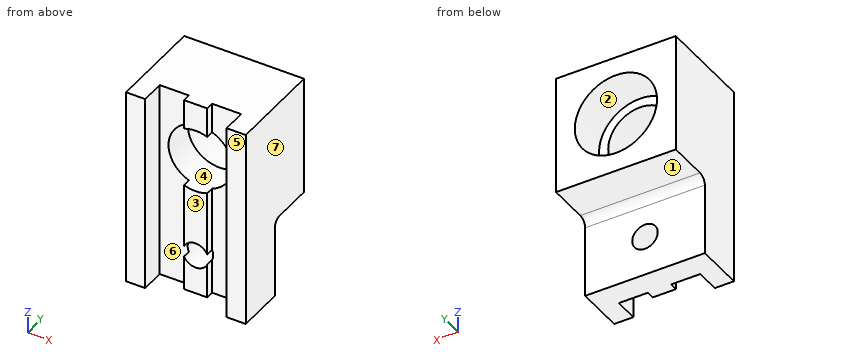
from build123d import *

# Parameters (mm, degrees)
MAIN_DEPTH         = 25
SKETCH2_R          = 5.15
ROLLINGHOLE_DEPTH  = 5
SKETCH3_R          = 4
CUT_EXTRUDE2_DEPTH = 8
SKETCH4_R          = 1.6
FIXHOLE_DEPTH      = 13
SKETCH5_W          = 10
SKETCH5_H          = 6
CUT_EXTRUDE4_DEPTH = 16
FILLET1_R          = 1


with BuildPart() as part:
    # Sketch1 → Main (new body)
    with BuildSketch(Plane.XY):
        Polygon((-5.1, 0), (-5.1, -3), (-7.5, -3), (-7.5, 9), (7.5, 9), (7.5, -3), (5.1, -3), (5.1, 0), (1.45, 0), (1.45, -1), (-1.45, -1), (-1.45, 0), align=None)
    extrude(amount=MAIN_DEPTH)

    # Sketch2 → RollingHole (cut)
    with BuildSketch(Plane(origin=(0, 9, 0), x_dir=(1, 0, 0), z_dir=(0, 1, 0))):
        with Locations((0, -17.5)):
            Circle(SKETCH2_R)
    extrude(amount=-ROLLINGHOLE_DEPTH, mode=Mode.SUBTRACT)

    # Sketch3 → Cut-Extrude2 (cut, through all)
    with BuildSketch(Plane(origin=(0, 4, 0), x_dir=(1, 0, 0), z_dir=(0, 1, 0))):
        with Locations((0, -17.5)):
            Circle(SKETCH3_R)
    extrude(amount=-CUT_EXTRUDE2_DEPTH, mode=Mode.SUBTRACT)

    # Sketch4 → FixHole (cut, through all)
    with BuildSketch(Plane(origin=(0, 9, 0), x_dir=(1, 0, 0), z_dir=(0, 1, 0))):
        with Locations((0, -5)):
            Circle(SKETCH4_R)
    extrude(amount=-FIXHOLE_DEPTH, mode=Mode.SUBTRACT)

    # Sketch5 → Cut-Extrude4 (cut, through all)
    with BuildSketch(Plane.ZY.offset(7.5)):
        with Locations((5, 6)):
            Rectangle(SKETCH5_W, SKETCH5_H)
    extrude(amount=-CUT_EXTRUDE4_DEPTH, mode=Mode.SUBTRACT)

    # Fillet1
    fillet1_edges = [part.edges().sort_by_distance(p)[0] for p in [
        (0, 3, 10),
    ]]
    fillet(fillet1_edges, radius=FILLET1_R)


solid = part.part
Check sheet for the modelled part. Datum: model origin and axes. Units: mm. Face numbers are marked on the shaded views. A direction names the side the tool comes from. Round coordinates to 2 decimals unless told otherwise and drop trailing zeros. Order: outer loops, then holes, each group sorted by start corner. A loop starts at its lowest first (then second) coordinate and runs counter-clockwise, first axis right, second up. Notation, with made-up numbers: M -33.5,19 L 8.5,19 A25 cw 8.5,45 Z; hole C 4,85.5 d2. An arc over 180 degrees is marked long. One line per item, written item: value. Start each with the question number.
1. Section check C-C on x = 0. Enter the section's corners in (y, z), and give its area (3 significant figures).
2. Access from +Z, -Z, +X, -X, +Y, -Y to the whole of each face (thin tool, end or side, straight path). Record for the marked faces 1, 2, 3 and 4.
3. Section check B-B on z = 17.5. Enter the section's corners in (x, y).
4. Release check for a two-part mould opening along X. For the marked faces 5, 6 and 7 record: released by +X, released by -X, zero draft, split by the parting line, or undercut.
5. Section check D-D on y = 6.5. Enter the section's corners in (x, z).
6. Section check A-A on y = -0.5. Enter the section's corners in (x, z).
7. Gauge pin test, flat ends, axial feed: P1, Ø1.5, axis at x = 0, z = 22.5, coming from the -Y side; P2, Ø1.5, axis at x = -4.5, z = 9, coming from the +Y side; P3, Ø4, axis at x = 0, z = 5, coming from the +Y side. Record the tip position at first contact, or that the pin passes through.
8. Scan lines: line 1 along Z through (x, y) = (0, 0.6); line 2 along X through (y, z) = (0.4, 5); line 3 along X through (y, z) = (2.65, 17.5). Record each from-to range of solid material in increasing order.
Results found:
1. outline: M -1,0 L 3,0 L 3,3.4 L -1,3.4 Z; M -1,6.6 L 3,6.6 L 3,9 A1 cw 4,10 L 9,10 L 9,12.35 L 4,12.35 L 4,13.5 L -1,13.5 Z; M -1,21.5 L 4,21.5 L 4,22.65 L 9,22.65 L 9,25 L -1,25 Z
1. area: 85.9 mm^2
2. face 1: -Z, +X, -X, +Y
2. face 2: +Y
2. face 3: +Z, -Z, -Y
2. face 4: +Y, -Y
3. outline: M -7.5,-3 L -5.1,-3 L -5.1,0 L -4,0 L -4,4 L -5.15,4 L -5.15,9 L -7.5,9 Z; M 4,0 L 5.1,0 L 5.1,-3 L 7.5,-3 L 7.5,9 L 5.15,9 L 5.15,4 L 4,4 Z
4. face 5: zero draft
4. face 6: undercut
4. face 7: released by +X
5. outline: M -7.5,10 L 7.5,10 L 7.5,25 L -7.5,25 Z; hole C 0,17.5 d10.3
6. outline: M -7.5,0 L -5.1,0 L -5.1,25 L -7.5,25 Z; M -1.45,0 L 1.45,0 L 1.45,4.32 A1.6 cw -1.45,4.32 Z; M -1.45,5.68 A1.6 cw 1.45,5.68 L 1.45,13.77 A4 cw -1.45,13.77 Z; M -1.45,21.23 A4 cw 1.45,21.23 L 1.45,25 L -1.45,25 Z; M 5.1,0 L 7.5,0 L 7.5,25 L 5.1,25 Z
7. P1: y = -1
7. P2: y = 3.34
7. P3: y = 3
8. line 1: 0 to 3.4, 6.6 to 13.5, 21.5 to 25
8. line 2: -7.5 to -1.6, 1.6 to 7.5
8. line 3: -7.5 to -4, 4 to 7.5
